from build123d import *

# Parameters (mm, degrees)
F0_W     = 30
F0_H     = 45
F1_DEPTH = 2
F3_D     = 2
F4_D     = 3
F2_W     = 3
F2_H     = 8.5
F5_DEPTH = 19
F6_SIZE2 = 18.99999
F6_SIZE  = 7.99999


# Not quite as in the source:
# - a fillet or chamfer is up to 0.001 mm smaller than in the source, because OpenCascade refuses the exact size


with BuildPart() as f1:
    # F0 (on Front) → F1 (new body)
    with BuildSketch(Plane.XZ):
        Rectangle(F0_W, F0_H)
    extrude(amount=F1_DEPTH)

    # F3 (through all)
    with Locations(Plane.XZ.offset(2)):
        with Locations((-7, 20.5), (7, 20.5)):
            Hole(F3_D / 2)

    # F4 (through all)
    with Locations(Plane.XZ.offset(2)):
        with Locations((0, 7.5), (0, -7.5)):
            Hole(F4_D / 2)

    # F2 (on face) → F5 (join)
    with BuildSketch(Plane.XZ.offset(2)):
        with Locations((0, 14.75)):
            Rectangle(F2_W, F2_H)
    extrude(amount=F5_DEPTH)

    # F6 (size 8 and 19 in the source; OpenCascade refuses exactly that, so slightly less here)
    f6_edges = [f1.edges().sort_by_distance(p)[0] for p in [
        (0, -21, 10.5),
    ]]
    f6_side = f1.faces().sort_by_distance((0, -21, 14.75))[0]
    chamfer(f6_edges, length=F6_SIZE, length2=F6_SIZE2, reference=f6_side)


solid = f1.part
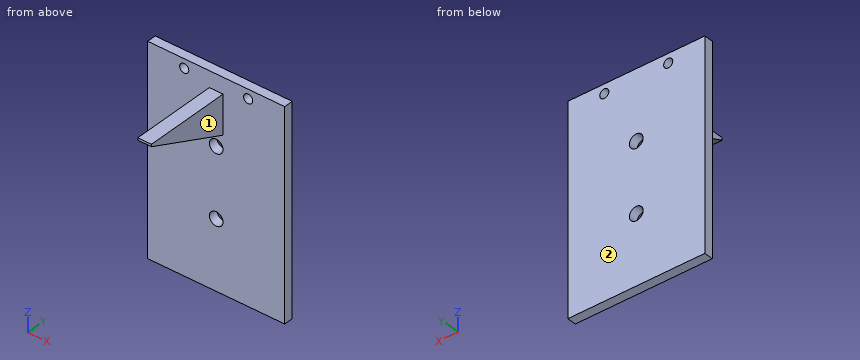
Design review of the part built by this model. Coordinates are the model's own, in mm. Face numbers are marked on the shaded views. A direction names the side the tool comes from. Round coordinates to 2 decimals unless told otherwise and drop trailing zeros. Order: outer loops, then holes, each group sorted by start corner. A loop starts at its lowest first (then second) coordinate and runs counter-clockwise, first axis right, second up.
1) Clearance check with flat-ended pins moving along their axes: pin 1 Ø2.5 at (x, z) = (0, 7.5) entering from -Y; pin 2 Ø2 at (x, y) = (-2, -5) entering from +Z; pin 3 Ø5 at (x, z) = (4.5, 11) entering from -Y; pin 4 Ø2.5 at (y, z) = (-7.5, 13.5) entering from -X. State where each tip first meets the part, or that it passes through.
The answers:
pin 1: passes through
pin 2: stops at z = 19
pin 3: stops at y = -2
pin 4: stops at x = -1.5
2) Consider section D-D (z = 12). State the section outline as (x, y) points.
The answers:
outline: (-15, -2) - (-1.5, -2) - (-1.5, -5.56) - (1.5, -5.56) - (1.5, -2) - (15, -2) - (15, 0) - (-15, 0) - close
3) Consider section A-A (x = 7). State the section outline as (y, z) points.
The answers:
outline: (-2, -22.5) - (0, -22.5) - (0, 19.5) - (-2, 19.5) - close; (-2, 21.5) - (0, 21.5) - (0, 22.5) - (-2, 22.5) - close
4) Machinability: for the marked faces 1 and 2, which of the approach directions +Z, -Z, +X, -X, +Y, -Y give a long, thin tool a straight path to every point of the face, cutting with its end or side? Answer none if there is none.
The answers:
face 1: +Z, -Z, +X, -Y
face 2: +Z, -Z, +X, -X, +Y
5) For L1, parallel to Z at x = 0, y = -1.15; L2, parallel to Z at x = -7, y = -1.1; L3, parallel to Y at x = -2.5, z = 10, list the stretches that pass through material, from the lowest coordinate up.
The answers:
L1: z = -22.5 to -9, -6 to 6, 9 to 22.5
L2: z = -22.5 to 19.5, 21.5 to 22.5
L3: y = -2 to 0
6) Consider section B-B (z = -7.5). State the section outline as (x, y) points, plus the area to 3 significant figures.
The answers:
outline: (-15, -2) - (-1.5, -2) - (-1.5, 0) - (-15, 0) - close; (1.5, -2) - (15, -2) - (15, 0) - (1.5, 0) - close
area: 54.0 mm2
7) Consider section C-C (z = 20.5). State the section outline as (x, y) points, plus the area to 3 significant figures.
The answers:
outline: (-15, -2) - (-8, -2) - (-8, 0) - (-15, 0) - close; (-6, -2) - (6, -2) - (6, 0) - (-6, 0) - close; (8, -2) - (15, -2) - (15, 0) - (8, 0) - close
area: 52.0 mm2
